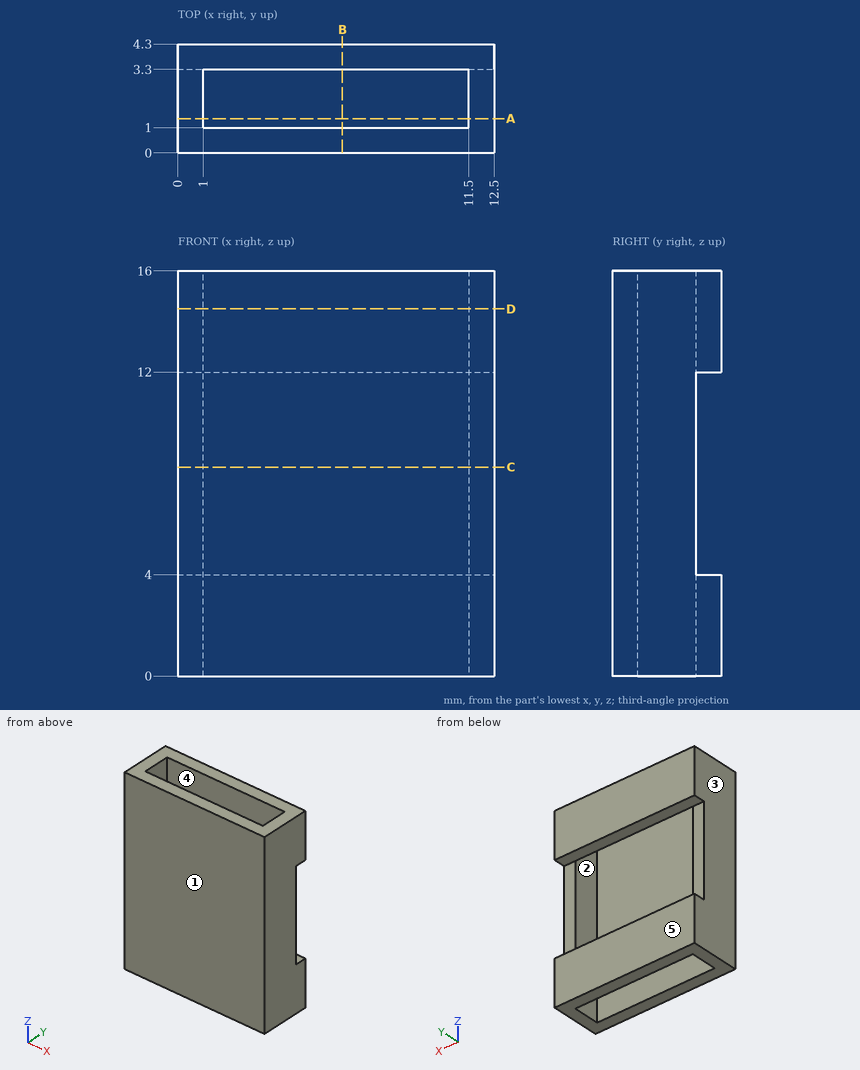
Here's the drawing with two shaded views (mm, measured from the low corner). I have some questions. A direction names the side the tool comes from. Coordinates: 2 decimals unless noted, no trailing zeros. Write each loop counter-clockwise with the first axis right and the second up, starting at its lowest first coordinate (ties: lowest second). Pieces come first, ordered by that corner, then holes. Notation, with made-up numbers: M -7.75,-33.75 L 21.25,-33.75 A32 cw 21.25,-0.75 Z; hole C 27.25,69.5 d11. An arc over 180 degrees is marked long. Use one line per item in the form item = value.
Q1. If we section it at C-C (z = 8.25): Write out the boundary of the cut face in (x, y), then the cut area to 3 significant figures.
Model answer:
outline = M 0,0 L 12.5,0 L 12.5,3.3 L 11.5,3.3 L 11.5,1 L 1,1 L 1,3.3 L 0,3.3 Z
area = 17.1 mm^2
Q2. We'd pull the mould along X, two halves only. Please class the marked faces 1, 2 and 3: +X half, -X half, draft (parallel to the pull), parting line (faces both ways), or undercut.
Model answer:
face_1 = draft
face_2 = undercut
face_3 = -X half
Q3. If we section it at D-D (z = 14.5): Write out the boundary of the cut face in (x, y), then the cut area to 3 significant figures.
Model answer:
outline = M 0,0 L 12.5,0 L 12.5,4.3 L 0,4.3 Z; hole M 1,1 L 11.5,1 L 11.5,3.3 L 1,3.3 Z
area = 29.6 mm^2
Q4. If we section it at A-A (y = 1.35): Write out the boundary of the cut face in (x, z), then the cut area to 3 significant figures.
Model answer:
outline = M 0,0 L 1,0 L 1,16 L 0,16 Z; M 11.5,0 L 12.5,0 L 12.5,16 L 11.5,16 Z
area = 32.0 mm^2
Q5. For P1, Ø4, axis at x = 9.5, z = 9, coming from the -Y side; P2, Ø0.8, axis at x = 0.5, z = 9.5, coming from the +Y side; P3, Ø1.5, axis at x = 2.5, y = 2, coming from the -Z side, each with a flat end and sliding along its axis, tell me the tip position at first contact or that it passes through.
Model answer:
P1 = 0
P2 = 3.3
P3 = through
Q6. For the marked faces 4 and 5, which set-ups out of +Z, -Z, +X, -X, +Y, -Y let a thin tool reach every point of the face, with its end or its side?
Model answer:
face_4 = +Z, -Z
face_5 = +Z, -Z, +X, -X, +Y
Q7. If we section it at B-B (x = 6.5): Write out the boundary of the cut face in (y, z).
Model answer:
outline = M 0,0 L 1,0 L 1,16 L 0,16 Z; M 3.3,0 L 4.3,0 L 4.3,4 L 3.3,4 Z; M 3.3,12 L 4.3,12 L 4.3,16 L 3.3,16 Z
Q8. I need wall thicknesses on line 1 along X through (y, z) = (2.1, 8.25); line 2 along Y through (x, z) = (2.5, 12.75); line 3 along Z through (x, y) = (11.75, 3.5). Which ranges of each line are inside material? Lowest first, please. Write a range as from..to.
Model answer:
line_1 = 0..1, 11.5..12.5
line_2 = 0..1, 3.3..4.3
line_3 = 0..4, 12..16
